from build123d import *

# Parameters (mm, degrees)
CROQUIS1_W              = 60
CROQUIS1_H              = 170
SALIENTE_EXTRUIR1_DEPTH = 5
CROQUIS2_W              = 10
CROQUIS2_H              = 10
SALIENTE_EXTRUIR2_DEPTH = 27.5
CROQUIS3_R              = 2.5
CORTAR_EXTRUIR1_DEPTH   = 27.5
CROQUIS4_W              = 2
CROQUIS4_H              = 25
CORTAR_EXTRUIR2_DEPTH   = 27.5
CROQUIS6_W              = 60
CROQUIS6_H              = 5
SALIENTE_EXTRUIR3_DEPTH = 10
CROQUIS7_W              = 2
CROQUIS7_H              = 25
CORTAR_EXTRUIR3_DEPTH   = 10


with BuildPart() as part:
    # Croquis1 → Saliente-Extruir1 (new body)
    with BuildSketch(Plane.XY):
        with Locations((30, 85)):
            Rectangle(CROQUIS1_W, CROQUIS1_H)
    extrude(amount=SALIENTE_EXTRUIR1_DEPTH)

    # Croquis2 → Saliente-Extruir2 (add)
    with BuildSketch(Plane.XY.offset(5)):
        with Locations((20, 100)):
            Rectangle(CROQUIS2_W, CROQUIS2_H)
        with Locations((5, 100)):
            Rectangle(CROQUIS2_W, CROQUIS2_H)
        with Locations((20, 25)):
            Rectangle(CROQUIS2_W, CROQUIS2_H)
        with Locations((5, 25)):
            Rectangle(CROQUIS2_W, CROQUIS2_H)
    extrude(amount=SALIENTE_EXTRUIR2_DEPTH)

    # Croquis3 → Cortar-Extruir1 (cut)
    with BuildSketch(Plane(origin=(25, 0, 0), x_dir=(0, 0, -1), z_dir=(1, 0, 0))):
        with Locations((-27.5, 100)):
            Circle(CROQUIS3_R)
        with Locations((-10, 100)):
            Circle(CROQUIS3_R)
        with Locations((-27.5, 25)):
            Circle(CROQUIS3_R)
        with Locations((-10, 25)):
            Circle(CROQUIS3_R)
    extrude(amount=-CORTAR_EXTRUIR1_DEPTH, mode=Mode.SUBTRACT)

    # Croquis4 → Cortar-Extruir2 (cut)
    with BuildSketch(Plane.XY.offset(5)):
        with Locations((6, 150.5)):
            Rectangle(CROQUIS4_W, CROQUIS4_H)
        with Locations((54, 150.5)):
            Rectangle(CROQUIS4_W, CROQUIS4_H)
    extrude(amount=-CORTAR_EXTRUIR2_DEPTH, mode=Mode.SUBTRACT)

    # Croquis6 → Saliente-Extruir3 (add)
    with BuildSketch(Plane.XZ):
        with Locations((30, 2.5)):
            Rectangle(CROQUIS6_W, CROQUIS6_H)
    extrude(amount=SALIENTE_EXTRUIR3_DEPTH)

    # Croquis7 → Cortar-Extruir3 (cut)
    with BuildSketch(Plane.XY.offset(5)):
        with Locations((6, 7.5)):
            Rectangle(CROQUIS7_W, CROQUIS7_H)
        with Locations((54, 7.5)):
            Rectangle(CROQUIS7_W, CROQUIS7_H)
    extrude(amount=-CORTAR_EXTRUIR3_DEPTH, mode=Mode.SUBTRACT)


solid = part.part
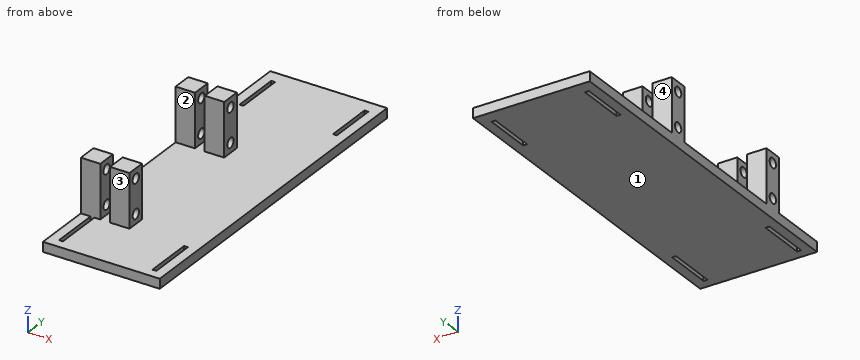
Read the model definition and answer for the solid it produces. Units are mm, in the model's axes. Face numbers are marked on the shaded views. Round coordinates to 2 decimals unless told otherwise and drop trailing zeros. Loops run counter-clockwise (first coordinate to the right, second up) from the corner with the lowest first, then second, coordinate; pieces in that order, holes last.
Q1. Consider probe 1 along Y at (x, z) = (5.25, 27.5); probe 2 along Y at (x, z) = (22.5, 6); probe 3 along X at (y, z) = (29, 14.5). Determine where each line is inside the solid, lowest interval first.
Q2. Section B-B on y = 25 is taken. Write down the section's boundary in (x, z).
Q3. Section A-A on z = 27.5 is taken. Give the number of separate pieces and of enclosed holes in the cut face, and give its area (3 significant figures).
Q4. Section C-C on z = 3 is taken. Write down the section's boundary in (x, y).
Q5. Determine the mould class of the marked faces 1, 2, 3 and 4 for opening direction Y: released by +Y, released by -Y, zero draft, split by the parting line, or undercut.
Q6. Each of these flat-tipped pins is pushed along its axis until it touches: pin 1 (3 mm diameter, centred on y = 97.5, z = 17.5, fed in from +X); pin 2 (8 mm diameter, centred on x = 10, y = 86, fed in from -Z); pin 3 (4 mm diameter, centred on y = 100, z = 27.5, fed in from +X); pin 4 (5 mm diameter, centred on x = 4.5, z = 20.5, fed in from -Y). Where does it stop, or does it pass through?
Q7. Section D-D on y = 145 is taken. Write down the section's boundary in (x, z).
Output:
1. probe 1: y = 20 to 22.5, 27.5 to 30, 95 to 97.5, 102.5 to 105
1. probe 2: y = 20 to 30, 95 to 105
1. probe 3: x = 0 to 10, 15 to 25
2. outline: (0, 0) - (60, 0) - (60, 5) - (25, 5) - (25, 7.5) - (15, 7.5) - (15, 5) - (10, 5) - (10, 7.5) - (0, 7.5) - close; (0, 12.5) - (10, 12.5) - (10, 25) - (0, 25) - close; (0, 30) - (10, 30) - (10, 32.5) - (0, 32.5) - close; (15, 12.5) - (25, 12.5) - (25, 25) - (15, 25) - close; (15, 30) - (25, 30) - (25, 32.5) - (15, 32.5) - close
3. separate pieces: 8
3. enclosed holes: 0
3. area: 200 mm2
4. outline: (0, -10) - (60, -10) - (60, 170) - (0, 170) - close; hole (5, -5) - (7, -5) - (7, 20) - (5, 20) - close; hole (5, 138) - (7, 138) - (7, 163) - (5, 163) - close; hole (53, -5) - (55, -5) - (55, 20) - (53, 20) - close; hole (53, 138) - (55, 138) - (55, 163) - (53, 163) - close
5. face 1: zero draft
5. face 2: undercut
5. face 3: released by -Y
5. face 4: released by +Y
6. pin 1: stops at x = 25
6. pin 2: stops at z = 0
6. pin 3: passes through
6. pin 4: stops at y = 20
7. outline: (0, 0) - (5, 0) - (5, 5) - (0, 5) - close; (7, 0) - (53, 0) - (53, 5) - (7, 5) - close; (55, 0) - (60, 0) - (60, 5) - (55, 5) - close
